Verification items for this drawing (mm, ordinates from the low corner). A direction names the side the tool comes from. Give positions to 0.01 mm unless a question says otherwise; leave off trailing zeros. Write each loop counter-clockwise with the first axis right and the second up, starting at its lowest first coordinate (ties: lowest second). Pieces come first, ordered by that corner, then holes. Notation, with made-up numbers: M 11,2 L 62,2 A21 cw 62,35 Z; hole C 81.5,38.5 d8. An arc over 180 degrees is marked long. Use one line per item in the form item = value. Start each with the question number.
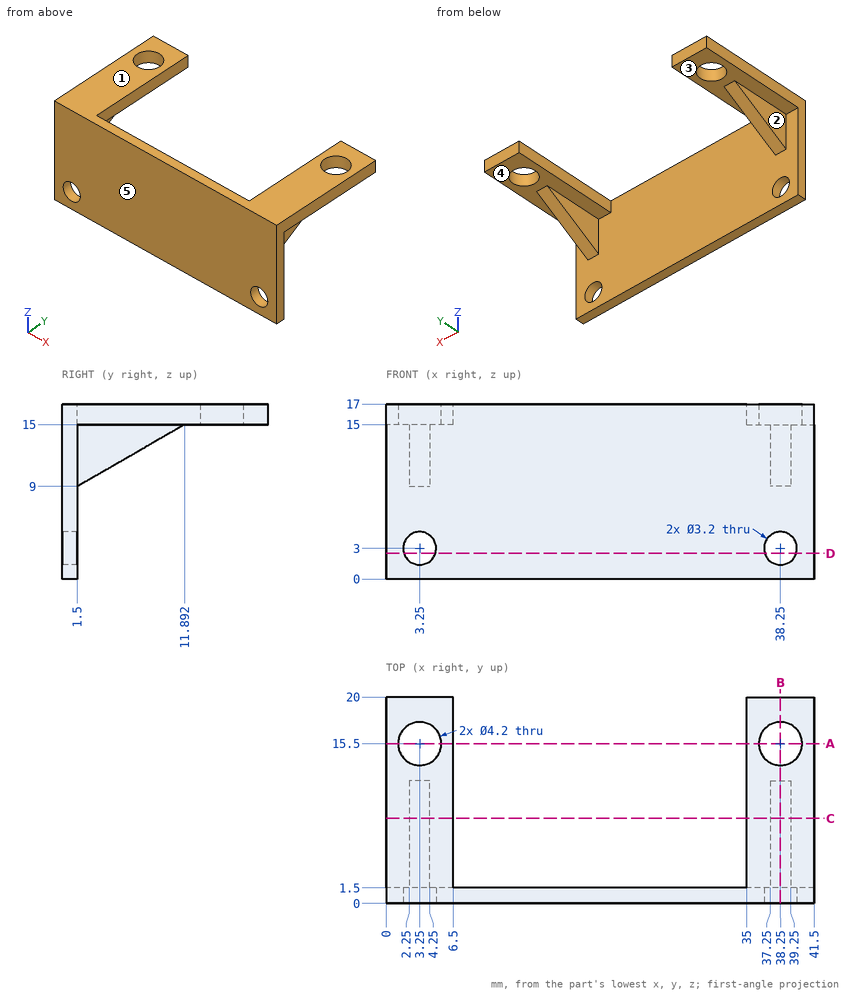
(1) Depth check by flat-ended pin: pin 1 (5 mm diameter, centred on y = 6, z = 11, fed in from +X); pin 2 (2 mm diameter, centred on x = 37.5, y = 6.5, fed in from -Z); pin 3 (3.5 mm diameter, centred on x = 3.25, y = 15.5, fed in from -Z); pin 4 (8.5 mm diameter, centred on x = 24, z = 8, fed in from +Y). Enter the tip coordinate at first touch or a pass-through.
(2) Sectioned sample at A-A, the plane y = 15.5. Record the boundary of the cut face in (x, z).
(3) Tool access check on the marked faces 4 and 5. Record the directions out of +Z, -Z, +X, -X, +Y, -Y that give a thin tool (end or side, any length) a straight path to the whole face; none if there is none.
(4) Sectioned sample at C-C, the plane y = 8.25. Record the boundary of the cut face in (x, z).
(5) Thickness scan on probe 1 along X at (y, z) = (0.85, 3); probe 2 along Z at (x, y) = (3.25, 0.7); probe 3 along Y at (x, z) = (3.25, 16.45). Record the ranges inside material, lowest first. Write a range as [from, to].
(6) Sectioned sample at D-D, the plane z = 2.5. Record the boundary of the cut face in (x, y).
(7) Sectioned sample at B-B, the plane x = 38.25. Record the boundary of the cut face in (y, z).
(8) Draft check along X on the marked faces 1, 2 and 3. Enter one of: released by +X, released by -X, zero draft, split by the parting line, or undercut.
Numbers:
q1.pin_1 = 39.25
q1.pin_2 = 11.31
q1.pin_3 = through
q1.pin_4 = 1.5
q2.outline = M 0,15 L 1.15,15 L 1.15,17 L 0,17 Z; M 5.35,15 L 6.5,15 L 6.5,17 L 5.35,17 Z; M 35,15 L 36.15,15 L 36.15,17 L 35,17 Z; M 40.35,15 L 41.5,15 L 41.5,17 L 40.35,17 Z
q3.face_4 = -Z, +Y
q3.face_5 = +Z, -Z, +X, -X, -Y
q4.outline = M 0,15 L 2.25,15 L 2.25,12.9 L 4.25,12.9 L 4.25,15 L 6.5,15 L 6.5,17 L 0,17 Z; M 35,15 L 37.25,15 L 37.25,12.9 L 39.25,12.9 L 39.25,15 L 41.5,15 L 41.5,17 L 35,17 Z
q5.probe_1 = [0, 1.65], [4.85, 36.65], [39.85, 41.5]
q5.probe_2 = [0, 1.4], [4.6, 17]
q5.probe_3 = [0, 13.4], [17.6, 20]
q6.outline = M 0,0 L 1.73,0 L 1.73,1.5 L 0,1.5 Z; M 4.77,0 L 36.73,0 L 36.73,1.5 L 4.77,1.5 Z; M 39.77,0 L 41.5,0 L 41.5,1.5 L 39.77,1.5 Z
q7.outline = M 0,0 L 1.5,0 L 1.5,1.4 L 0,1.4 Z; M 0,4.6 L 1.5,4.6 L 1.5,9 L 11.89,15 L 13.4,15 L 13.4,17 L 0,17 Z; M 17.6,15 L 20,15 L 20,17 L 17.6,17 Z
q8.face_1 = zero draft
q8.face_2 = released by -X
q8.face_3 = undercut
